Read the model definition and answer for the solid it produces. Units are mm, in the model's axes. A direction names the side the tool comes from. Coordinates: 2 decimals unless noted, no trailing zeros. Write each loop counter-clockwise with the first axis right and the second up, starting at its lowest first coordinate (ties: lowest second). Pieces come first, ordered by that corner, then holes. Notation, with made-up numbers: (11, 60) -> (18, 60) arc R29 cw to (18, 97) -> close; hole circle Ø11 at (51.5, 10). An arc over 180 degrees is marked (long way). One line per item, written item: value. Start each with the question number.
1. Find section D-D, the plane y = 2. Write down the section's boundary in (x, z), and give its area (3 significant figures).
2. For a pull along X with two mould halves and no side action, classify faces 4 (the flat face through (115, -21, 0)), 5 (the flat face through (135, 0, 0)), 6 (the cylindrical face through (118.726, -12.686, 5.059)) as pulls with the +X half, pulls with the -X half, needs draft (parallel to the pull), parting line crosses it, or undercut.
3. Find section A-A, the plane y = -16.75. Write down the section's boundary in (x, z).
4. Given P1, Ø1.5, axis at y = -14.5, z = -3.5, coming from the +X side; P2, Ø1, axis at x = 97.5, z = -3, coming from the -Y side; P3, Ø12, axis at x = 100.5, y = -11.5, coming from the +Z side, each flat-ended and moving along its own axis, determine where each tip first touches the part or whether it passes through.
5. Find section B-B, the plane z = 0. Write down the section's boundary in (x, y), and give its area (3 significant figures).
6. Consider line 1 along Y through (x, z) = (27, 0.25); line 2 along X through (y, z) = (-10.5, 1.25); line 3 along X through (y, z) = (-4.25, -5). Determine where each line is inside the solid, lowest interval first.
7. For faces 1 (the cylindrical face through (22.726, -12.686, 5.059)), 2 (the flat face through (19, -21, 0)), 3 (the cylindrical face through (68, 6, 0)), determine the directions among +Z, -Z, +X, -X, +Y, -Y from which every point of the face is accessible in a straight line to the end or side of a thin tool.
8. Find section C-C, the plane x = 19.5. Write down the section's boundary in (y, z), and give its area (3 significant figures).
```python
from build123d import *

# Parameters (mm, degrees)
SKETCH_W    = 135
SKETCH_H    = 6
SKETCH001_R = 6
PAD_DEPTH   = 21


with BuildPart() as part:
    # Sketch → Revolution (revolve)
    with BuildSketch(Plane.XY):
        with Locations((67.5, -3)):
            Rectangle(SKETCH_W, SKETCH_H)
    revolve(axis=Axis((0, 0, 0), (1, 0, 0)))

    # Sketch001 → Pad (new body)
    with BuildSketch(Plane.XZ):
        with Locations((19.5, 0)):
            Circle(SKETCH001_R)
        with Locations((115.5, 0)):
            Circle(SKETCH001_R)
    extrude(amount=PAD_DEPTH)


solid = part.part
```
Answer block:
1. outline: (0, -5.66) -> (135, -5.66) -> (135, 5.66) -> (0, 5.66) -> close
1. area: 1,530 mm2
2. face 4: needs draft
2. face 5: pulls with the +X half
2. face 6: undercut
3. outline: circle Ø12 at (19.5, 0); circle Ø12 at (115.5, 0)
4. P1: stops at x = 120.83
4. P2: stops at y = -5.45
4. P3: stops at z = 2.4
5. outline: (0, -6) -> (13.5, -6) -> (13.5, -21) -> (25.5, -21) -> (25.5, -6) -> (109.5, -6) -> (109.5, -21) -> (121.5, -21) -> (121.5, -6) -> (135, -6) -> (135, 6) -> (0, 6) -> close
5. area: 1,980 mm2
6. line 1: y = -5.99 to 5.99
6. line 2: x = 13.63 to 25.37, 109.63 to 121.37
6. line 3: x = 16.18 to 22.82, 112.18 to 118.82
7. face 1: -Y
7. face 2: +Z, -Z, +X, -X, -Y
7. face 3: none
8. outline: (-21, -6) -> (0, -6) arc R6 ccw to (0, 6) -> (-21, 6) -> close
8. area: 309 mm2
